Source: three-view drawing plus pictorial views. Frame: mm from the lowest corner of the part. Round coordinates to 2 decimals unless told otherwise and drop trailing zeros. Loops run counter-clockwise (first coordinate to the right, second up) from the corner with the lowest first, then second, coordinate; pieces in that order, holes last. Notation, with made-up numbers: (48, 70.25) -> (85, 70.25) arc R19 ccw to (85, 93.25) -> close; hole circle Ø11 at (83, 8). An arc over 180 degrees is marked (long way). Answer in a Markdown table with one row per item. Add a question column.
Q1. Section A-A, the plane y = 25.4. Output: boundary loops of the cut face in (x, z), and give its area (3 significant figures).
Q2. Pin query (flat end, axial travel): pin 1 (5 mm diameter, centred on x = 34.5, z = 7.5, fed in from -Y); pin 2 (1.5 mm diameter, centred on x = 11.5, z = 6.5, fed in from +Y). Return the tip coordinate at first contact, or that it passes through.
Q3. Section D-D, the plane x = 45.5. Output: boundary loops of the cut face in (y, z), and give its area (3 significant figures).
Q4. Section C-C, the plane z = 1. Output: boundary loops of the cut face in (x, y).
Q5. Ray query, L1, parallel to Y at x = 25.4, z = 2.15; L2, parallel to Z at x = 18.5, y = 48; L3, parallel to Y at x = 32, z = 1. Return the intervals inside material, ascending. Write a range as from..to.
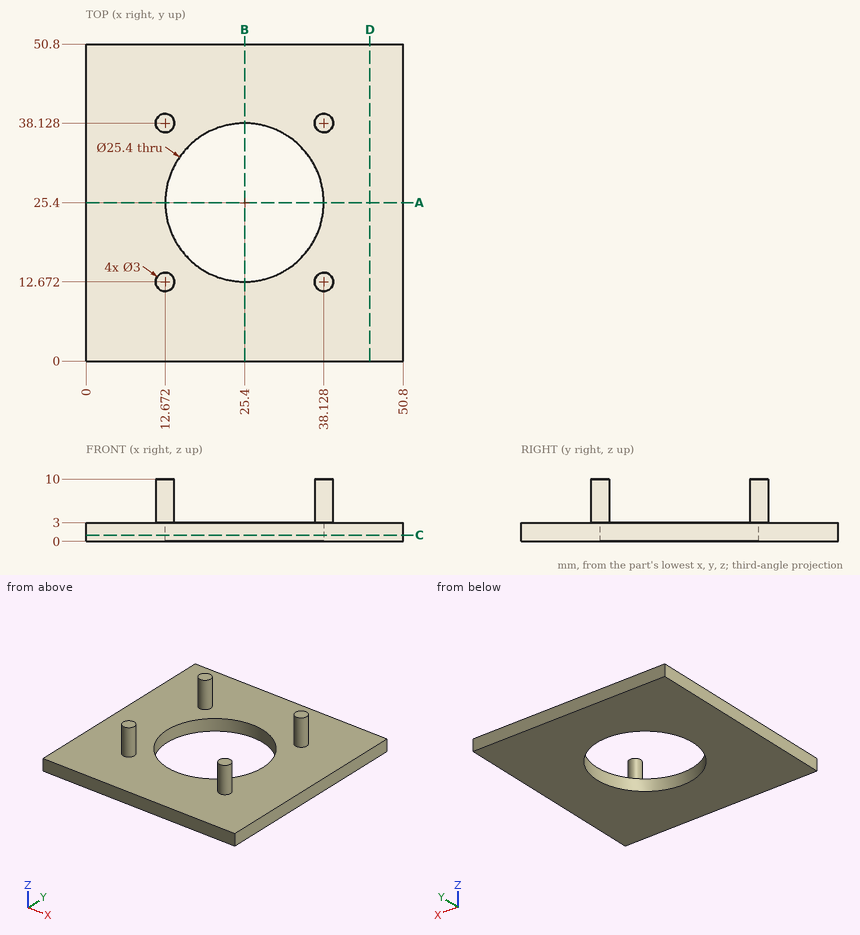
Answer block:
| question | item | result |
|---|---|---|
| 1 | outline | (0, 0) -> (12.7, 0) -> (12.7, 3) -> (0, 3) -> close; (38.1, 0) -> (50.8, 0) -> (50.8, 3) -> (38.1, 3) -> close |
| 1 | area | 76.2 mm^2 |
| 2 | pin 1 | y = 11.68 |
| 2 | pin 2 | y = 39.57 |
| 3 | outline | (0, 0) -> (50.8, 0) -> (50.8, 3) -> (0, 3) -> close |
| 3 | area | 152 mm^2 |
| 4 | outline | (0, 0) -> (50.8, 0) -> (50.8, 50.8) -> (0, 50.8) -> close; hole circle Ø25.4 at (25.4, 25.4) |
| 5 | L1 | 0..12.7, 38.1..50.8 |
| 5 | L2 | 0..3 |
| 5 | L3 | 0..14.55, 36.25..50.8 |
